```python
from build123d import *

# Parameters (mm, degrees)
CUT_EXTRUDE1_DEPTH      = 0.2
CUT_EXTRUDE1_DEPTH_BACK = 0.2
CUT_EXTRUDE2_DEPTH      = 0.2
CUT_EXTRUDE2_DEPTH_BACK = 0.2


with BuildPart() as part:
    # Sketch1 → Revolve1 (revolve)
    with BuildSketch(Plane.XY):
        with BuildLine():
            Line((-0.8, 0), (-0.8, 1.46601855))
            ThreePointArc((-0.8, 1.46601855), (-0.738085774, 1.679789478), (-0.571509952, 1.827383098))
            ThreePointArc((-0.571509952, 1.827383098), (-0.29223212, 1.93513645), (0, 2))
            Line((0, 2), (0, 1.25))
            Line((0, 1.25), (5.724, 1.25))
            Line((5.724, 1.25), (6, 0.974))
            Line((6, 0.974), (6, 0))
            Line((6, 0), (-0.8, 0))
        make_face()
    revolve(axis=Axis((6, 0, 0), (-1, 0, 0)))

    # Sketch2 → Cut-Extrude1 (cut, two sides)
    with BuildSketch(Plane.XY) as cut_extrude1_sk:
        with BuildLine():
            Line((-0.8, 1), (-0.8, -1))
            ThreePointArc((-0.8, -1), (-0.115415221, -0.639534952), (0.32, 0))
            ThreePointArc((0.32, 0), (-0.115415221, 0.639534952), (-0.8, 1))
        make_face()
    extrude(amount=CUT_EXTRUDE1_DEPTH, mode=Mode.SUBTRACT)
    extrude(cut_extrude1_sk.sketch, amount=-CUT_EXTRUDE1_DEPTH_BACK, mode=Mode.SUBTRACT)

    # Sketch3 → Cut-Extrude2 (cut, two sides)
    with BuildSketch(Plane(origin=(0, 0, 0), x_dir=(1, 0, 0), z_dir=(0, 1, 0))) as cut_extrude2_sk:
        with BuildLine():
            Line((-0.8, 1), (-0.8, -1))
            ThreePointArc((-0.8, -1), (-0.115415221, -0.639534952), (0.32, 0))
            ThreePointArc((0.32, 0), (-0.115415221, 0.639534952), (-0.8, 1))
        make_face()
    extrude(amount=CUT_EXTRUDE2_DEPTH, mode=Mode.SUBTRACT)
    extrude(cut_extrude2_sk.sketch, amount=-CUT_EXTRUDE2_DEPTH_BACK, mode=Mode.SUBTRACT)


solid = part.part
```
Part model, mm, in its own coordinate system. A direction names the side the tool comes from. Round coordinates to 2 decimals unless told otherwise and drop trailing zeros. Write each loop counter-clockwise with the first axis right and the second up, starting at its lowest first coordinate (ties: lowest second). Pieces come first, ordered by that corner, then holes. Notation, with made-up numbers: M 86.25,-28 L 121.25,-28 A6 ccw 121.25,-18 Z; hole C -8,65.5 d9. An arc over 180 degrees is marked long. One line per question, with ' | ' between items.
(1) Probe line 1 along Y through (x, z) = (3, -0.05); line 2 along X through (y, z) = (1.3, 0.55); line 3 along Y through (x, z) = (-0.25, 0.5). List the from-to ranges inside material, lowest first.
Answer key:
line 1: y = -1.25 to 1.25 | line 2: x = -0.8 to 0 | line 3: y = -1.88 to -0.2, 0.2 to 1.88
(2) Saw through at A-A on x = 4. Write the cut outline in (y, z), then the cut area to 3 significant figures.
Answer key:
outline: C 0,0 d2.5 | area: 4.91 mm^2
(3) Pin check, flat tips, straight feed: pin 1 (1 mm diameter, centred on x = 3, z = -1, fed in from +Y); pin 2 (0.9 mm diameter, centred on x = -0.5, y = 1, fed in from +Z); pin 3 (2 mm diameter, centred on x = 2, y = 0.5, fed in from +Z); pin 4 (2 mm diameter, centred on y = -1.5, z = 1, fed in from +X). Stop position of each tip, or through.
Answer key:
pin 1: stops at y = 1.15 | pin 2: stops at z = 1.85 | pin 3: stops at z = 1.25 | pin 4: stops at x = 6
(4) Two-plate mould, pull along Z, no slides. Class faces 3 (the face through (2.9, -0.27, 1.22)), 4 (the face through (6, 0, 0)), 5 (the face through (-0.4, 0.5, -0.2)): released by +Z, released by -Z, zero draft, split by the parting line, or undercut.
Answer key:
face 3: split by the parting line | face 4: zero draft | face 5: undercut
(5) 3-axis set-ups, long thin cutter, end or side, ignore diameter. For faces 1 (the face through (-0.21, -0.72, 0)), 2 (the face through (0, 1, -1)): which of +Z, -Z, +X, -X, +Y, -Y reach the whole face in a straight line?
Answer key:
face 1: -X | face 2: +X
